Geometry: final body of the model. Coordinates: model frame, mm. A direction names the side the tool comes from. Round coordinates to 2 decimals unless told otherwise and drop trailing zeros. Order: outer loops, then holes, each group sorted by start corner. A loop starts at its lowest first (then second) coordinate and runs counter-clockwise, first axis right, second up. Notation, with made-up numbers: (-21, 1) -> (-10, 1) arc R31 ccw to (-10, 27) -> close; hole circle Ø11 at (24, -20). An arc over 180 degrees is marked (long way). Put each result on its own line as item: value.
```python
from build123d import *

# Parameters (mm, degrees)
SKETCH_1_R      = 1.05
EXTRUDE_1_DEPTH = 2.9
EXTRUDE_2_DEPTH = 1.35
SKETCH_3_W      = 0.8
SKETCH_3_H      = 3.134296818
EXTRUDE_3_DEPTH = 0.25
EXTRUDE_4_DEPTH = 1.8


with BuildPart() as part:
    # 草图1 → 凸台-拉伸1 (new, symmetric)
    with BuildSketch(Plane.XY):
        Polygon((1.8, 0), (-1.8, 0), (-2.194296818, -0.394296818), (-4.305703182, -0.394296818), (-4.7, 0), (-6.4, 0), (-6.4, 6.165703182), (6.4, 6.165703182), (6.4, 0), (4.7, 0), (4.305703182, -0.394296818), (2.194296818, -0.394296818), align=None)
        with Locations((-3.25, 1.05)):
            Circle(SKETCH_1_R, mode=Mode.SUBTRACT)
        with Locations((3.25, 1.05)):
            Circle(SKETCH_1_R, mode=Mode.SUBTRACT)
    extrude(amount=EXTRUDE_1_DEPTH, both=True)

    # 草图2 → 凸台-拉伸2 (add, symmetric)
    with BuildSketch(Plane.XY):
        with BuildLine():
            Line((1.47, 6.165703182), (2.77, 6.165703182))
            ThreePointArc((2.77, 6.165703182), (2.12, 6.815703182), (1.47, 6.165703182))
        make_face()
    extrude(amount=EXTRUDE_2_DEPTH, both=True)

    # 草图3 → 凸台-拉伸3 (add, symmetric)
    with BuildSketch(Plane.XY):
        with Locations((5.1, -1.567148409)):
            Rectangle(SKETCH_3_W, SKETCH_3_H)
        with Locations((0, -1.567148409)):
            Rectangle(SKETCH_3_W, SKETCH_3_H)
        with Locations((-5.1, -1.567148409)):
            Rectangle(SKETCH_3_W, SKETCH_3_H)
    extrude(amount=EXTRUDE_3_DEPTH, both=True)

    # 草图4 → 凸台-拉伸4 (add, symmetric)
    with BuildSketch(Plane.XY):
        Polygon((-7.755801096, 10.305254362), (5.784060724, 6.165703182), (5.1, 6.165703182), (-7.810114206, 10.112721195), align=None)
    extrude(amount=EXTRUDE_4_DEPTH, both=True)


solid = part.part
```
1. Cut plane C-C on x = -3.25. Return loops of the section in (y, z), and give its area (3 significant figures).
Ans:
outline: (-0.39, -2.9) -> (0, -2.9) -> (0, 2.9) -> (-0.39, 2.9) -> close; (2.1, -2.9) -> (6.17, -2.9) -> (6.17, 2.9) -> (2.1, 2.9) -> close; (8.72, -1.8) -> (8.93, -1.8) -> (8.93, 1.8) -> (8.72, 1.8) -> close
area: 26.6 mm²
2. Contact query for flat-ended pins moving along their axis: P1, Ø0.5, axis at x = 5, z = -1.5, coming from the -Y side; P2, Ø2, axis at x = 1.5, y = 9, coming from the -Z side; P3, Ø0.6, axis at y = -1.5, z = 0, coming from the +X side; P4, Ø2.5, axis at x = -3, z = 1, coming from the -Y side. Output: stop coordinate, or through.
Ans:
P1: y = 0
P2: through
P3: x = 5.5
P4: y = -0.39
3. Cut plane A-A on z = -2.3. Return loops of the section in (x, y).
Ans:
outline: (-6.4, 0) -> (-4.7, 0) -> (-4.31, -0.39) -> (-2.19, -0.39) -> (-1.8, 0) -> (1.8, 0) -> (2.19, -0.39) -> (4.31, -0.39) -> (4.7, 0) -> (6.4, 0) -> (6.4, 6.17) -> (-6.4, 6.17) -> close; hole circle Ø2.1 at (-3.25, 1.05); hole circle Ø2.1 at (3.25, 1.05)
4. Material intervals for probe 1 along Y at (x, z) = (-3.25, 0.4); probe 2 along Y at (x, z) = (3.25, 0.65); probe 3 along Z at (x, y) = (2.25, 6.5), sorted ascending.
Ans:
probe 1: -0.39 to 0, 2.1 to 6.17, 8.72 to 8.93
probe 2: -0.39 to 0, 2.1 to 6.17, 6.73 to 6.94
probe 3: -1.35 to 1.35
5. Cut plane D-D on x = -1.5. Return loops of the section in (y, z).
Ans:
outline: (0, -2.9) -> (6.17, -2.9) -> (6.17, 2.9) -> (0, 2.9) -> close; (8.18, -1.8) -> (8.39, -1.8) -> (8.39, 1.8) -> (8.18, 1.8) -> close
6. Draft query along X for faces 3 (the face through (2.134, 6.816, 0.019)), 4 (the face through (-6.4, 3, 0)), 5 (the face through (-5, -2, 0.25)). Return one class per face: +X half, -X half, draft (parallel to the pull), parting line (faces both ways), or undercut.
Ans:
face 3: undercut
face 4: -X half
face 5: draft
7. Set-up query: faces 1 (the face through (6.4, 3, 0)), 2 (the face through (-1.26, 8.11, 0.03)). Return all of +Z, -Z, +X, -X, +Y, -Y with unobstructed straight access to the full face (end or side cutting, diameter ignored); none if empty.
Ans:
face 1: +Z, -Z, +X, +Y, -Y
face 2: +Z, -Z
8. Cut plane B-B on y = 1.05. Return loops of the section in (x, z), and give its area (3 significant figures).
Ans:
outline: (-6.4, -2.9) -> (-4.3, -2.9) -> (-4.3, 2.9) -> (-6.4, 2.9) -> close; (-2.2, -2.9) -> (2.2, -2.9) -> (2.2, 2.9) -> (-2.2, 2.9) -> close; (4.3, -2.9) -> (6.4, -2.9) -> (6.4, 2.9) -> (4.3, 2.9) -> close
area: 49.9 mm²
